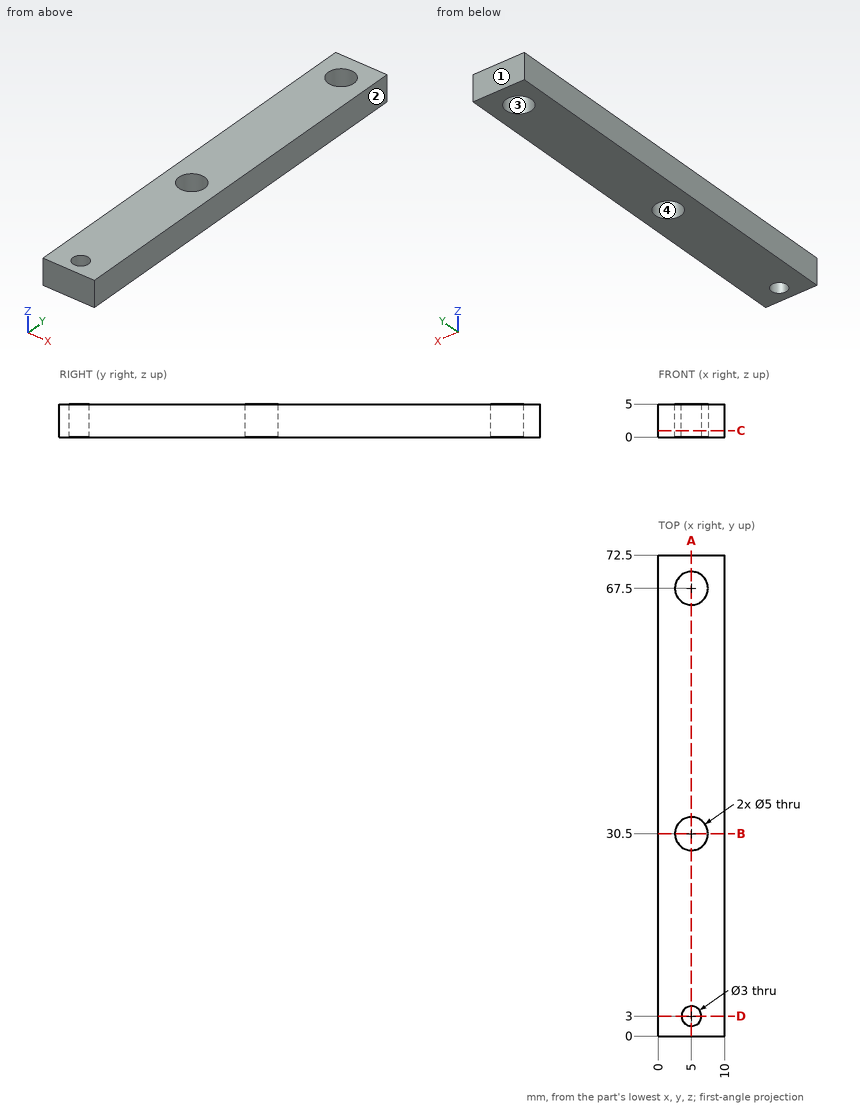
Geometry check sheet. Reference: drawing and pictorial views, mm from the part's lowest x, y, z. Give positions to 0.01 mm unless a question says otherwise; leave off trailing zeros. Loops run counter-clockwise (first coordinate to the right, second up) from the corner with the lowest first, then second, coordinate; pieces in that order, holes last. Notation, with made-up numbers: (47, 86.25) -> (86, 86.25) arc R30 ccw to (86, 124.25) -> close; hole circle Ø8 at (48, 42.5). An arc over 180 degrees is marked (long way). Answer in a Markdown table with one row per item. Add a question column.
1) Cross-section at B-B on y = 30.5. Record the boundary of the cut face in (x, z).
2) Cross-section at D-D on y = 3. Record the boundary of the cut face in (x, z), and give its area (3 significant figures).
3) Cross-section at C-C on z = 1. Record the boundary of the cut face in (x, y), and give its area (3 significant figures).
4) Cross-section at A-A on x = 5. Record the boundary of the cut face in (y, z).
5) Draft check along X on the marked faces 1, 2, 3 and 4. Enter one of: pulls with the +X half, pulls with the -X half, needs draft (parallel to the pull), parting line crosses it, or undercut.
6) Material ranges on probe 1 along Y at (x, z) = (5, 2.3); probe 2 along Y at (x, z) = (4.25, 3.95); probe 3 along X at (y, z) = (31, 2.45), recorded low to high. Write a range as from..to.
Outcome:
| question | item | result |
|---|---|---|
| 1 | outline | (0, 0) -> (2.5, 0) -> (2.5, 5) -> (0, 5) -> close; (7.5, 0) -> (10, 0) -> (10, 5) -> (7.5, 5) -> close |
| 2 | outline | (0, 0) -> (3.5, 0) -> (3.5, 5) -> (0, 5) -> close; (6.5, 0) -> (10, 0) -> (10, 5) -> (6.5, 5) -> close |
| 2 | area | 35.0 mm^2 |
| 3 | outline | (0, 0) -> (10, 0) -> (10, 72.5) -> (0, 72.5) -> close; hole circle Ø5 at (5, 30.5); hole circle Ø5 at (5, 67.5); hole circle Ø3 at (5, 3) |
| 3 | area | 679 mm^2 |
| 4 | outline | (0, 0) -> (1.5, 0) -> (1.5, 5) -> (0, 5) -> close; (4.5, 0) -> (28, 0) -> (28, 5) -> (4.5, 5) -> close; (33, 0) -> (65, 0) -> (65, 5) -> (33, 5) -> close; (70, 0) -> (72.5, 0) -> (72.5, 5) -> (70, 5) -> close |
| 5 | face 1 | needs draft |
| 5 | face 2 | pulls with the +X half |
| 5 | face 3 | undercut |
| 5 | face 4 | undercut |
| 6 | probe 1 | y = 0..1.5, 4.5..28, 33..65, 70..72.5 |
| 6 | probe 2 | y = 0..1.7, 4.3..28.12, 32.88..65.12, 69.88..72.5 |
| 6 | probe 3 | x = 0..2.55, 7.45..10 |
